Study the drawing (mm; zero at the part's minimum x, y, z) and answer. A direction names the side the tool comes from. Coordinates: 2 decimals unless noted, no trailing zeros. Loops run counter-clockwise (first coordinate to the right, second up) from the corner with the lowest first, then second, coordinate; pieces in that order, holes last.
Q1. Section D-D (y = 19) is taken. Give the vertices of the cut face in (x, z), then the cut area to 3 significant figures.
Q2. Section A-A (y = 4) is taken. Give the vertices of the cut face in (x, z).
Q3. Flat-ended cylindrical pins translate along their axes: P1, Ø1.2, axis at x = 9, y = 13, coming from the +Z side; P2, Ø5, axis at y = 18, z = 5, coming from the -X side; P3, Ø4.5, axis at y = 19.5, z = 7, coming from the +X side. Find the tip coordinate at first contact, or state that the pin passes through.
Q4. Straight lines are drawn through the part: line 1 (Y direction, x = 65, z = 8.2); line 2 (Y direction, x = 4, z = 8.85); line 3 (X direction, y = 3, z = 8.25). For each, find the intervals that lie inside material, in ascending order.
Q5. Section C-C (x = 58) is taken. Give the vertices of the cut face in (y, z), then the cut area to 3 significant figures.
Q6. Section B-B (z = 3) is taken. Give the vertices of the cut face in (x, y).
Q7. Which of the six approach directions +Z, -Z, +X, -X, +Y, -Y give full straight-line access (tool end or side, diameter ignored) to the marked faces 1, 2 and 3?
Q8. The mould has two halves that part along X. Classify the marked faces 4, 5 and 6: pulls with the +X half, pulls with the -X half, needs draft (parallel to the pull), parting line crosses it, or undercut.
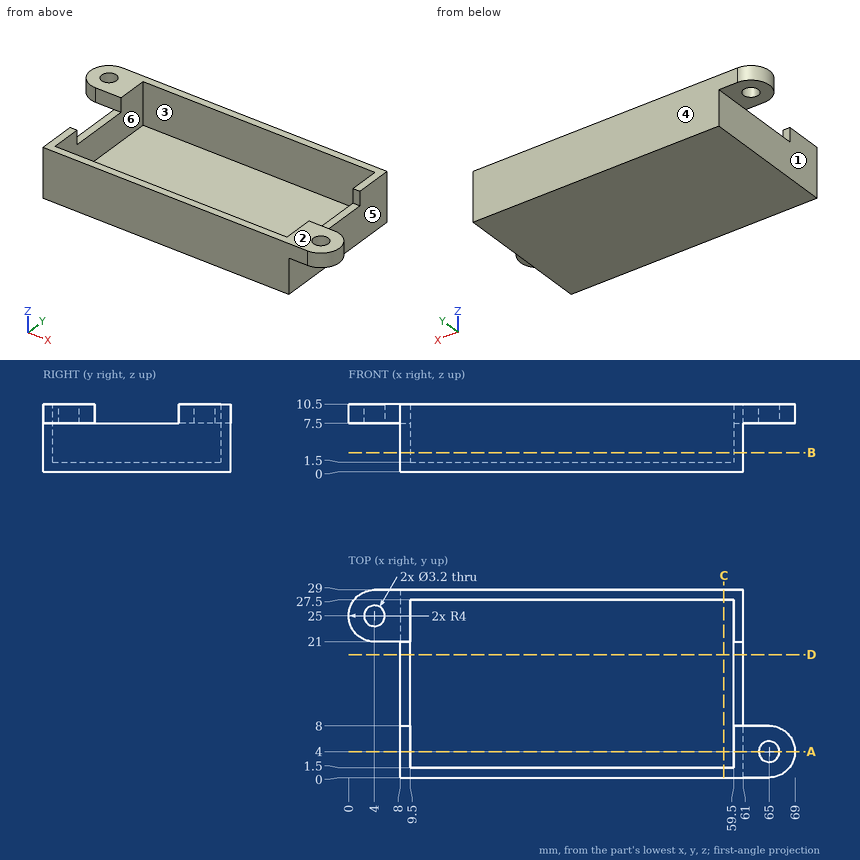
Numbers:
1. outline: (8, 0) - (61, 0) - (61, 7.5) - (59.5, 7.5) - (59.5, 1.5) - (9.5, 1.5) - (9.5, 7.5) - (8, 7.5) - close
1. area: 97.5 mm2
2. outline: (8, 0) - (61, 0) - (61, 7.5) - (63.4, 7.5) - (63.4, 10.5) - (59.5, 10.5) - (59.5, 1.5) - (9.5, 1.5) - (9.5, 10.5) - (8, 10.5) - close; (66.6, 7.5) - (69, 7.5) - (69, 10.5) - (66.6, 10.5) - close
3. P1: stops at z = 7.5
3. P2: stops at x = 8
3. P3: stops at x = 61
4. line 1: y = 0 to 2.4, 5.6 to 8
4. line 2: y = 21 to 23.4, 26.6 to 29
4. line 3: x = 8 to 9.5, 59.5 to 63.75, 66.25 to 68.87
5. outline: (0, 0) - (29, 0) - (29, 10.5) - (27.5, 10.5) - (27.5, 1.5) - (1.5, 1.5) - (1.5, 10.5) - (0, 10.5) - close
5. area: 70.5 mm2
6. outline: (8, 0) - (61, 0) - (61, 29) - (8, 29) - close; hole (9.5, 1.5) - (59.5, 1.5) - (59.5, 27.5) - (9.5, 27.5) - close
7. face 1: -Z, -X, -Y
7. face 2: +Z, +X, -X, +Y, -Y
7. face 3: +Z
8. face 4: needs draft
8. face 5: pulls with the +X half
8. face 6: undercut
